Geometry: final body of the model. Coordinates: model frame, mm. Face numbers are marked on the shaded views. A direction names the side the tool comes from. Coordinates: 2 decimals unless noted, no trailing zeros. Write each loop counter-clockwise with the first axis right and the second up, starting at its lowest first coordinate (ties: lowest second). Pieces come first, ordered by that corner, then holes. Notation, with made-up numbers: (63, 4) - (92, 4) arc R18 cw to (92, 8) - close; hole circle Ø5 at (57, -26). An arc over 180 degrees is marked (long way). Put each result on its own line as item: value.
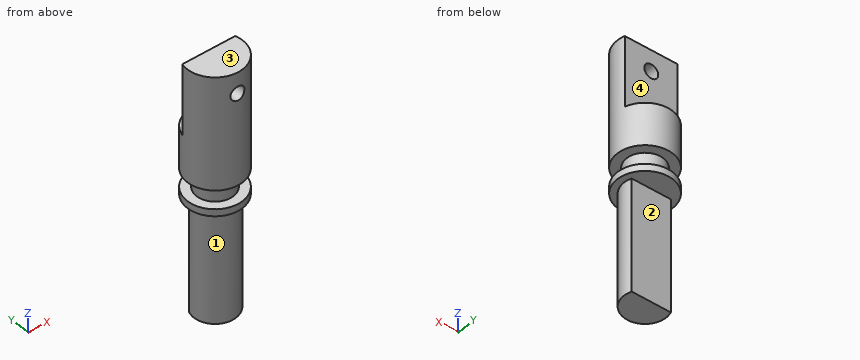
Autodesk Inventor part; units mm, degrees
ref_plane "YZ Plane" through (0, 0, 0) normal (1, 0, 0) x (0, 1, 0)
ref_plane "XZ Plane" through (0, 0, 0) normal (0, 1, 0) x (-1, 0, 0)
ref_plane "XY Plane" through (0, 0, 0) normal (0, 0, 1) x (1, 0, 0)
sketch "Sketch1" plane through (0, 0, 0) normal (0, 1, 0) x (-1, 0, 0)
  line L0 (0, 0) -> (-2.8001, 0)
  line L1 (-2.8001, 0) -> (-3.937, 0)
  line L2 (-3.937, 0) -> (-3.937, -16)
  line L3 (-3.937, -16) -> (-2.6225, -16)
  line L4 (-2.6225, -16) -> (-2.6225, -18.6416)
  line L5 (-2.6225, -18.6416) -> (-3.937, -18.6416)
  line L6 (-3.937, -18.6416) -> (-3.937, -19.6416)
  line L7 (-2.8001, 0) -> (0, 0)
  line L8 (-2.8001, 0) -> (0, 0)
  line L9 (-3.937, -19.6416) -> (-3, -19.6416)
  line L10 (-3, -19.6416) -> (-3, -35.6416)
  line L11 (-3, -35.6416) -> (0, -35.6416)
  line L12 (0, -35.6416) -> (0, 0)
  dimension "d1" = 0
  dimension "d2" = 16
  dimension "d3" = 2.6416
  dimension "d6" = 3.937
  dimension "d8" = 3
  dimension "d13" = 1
  dimension "d29" = 2.6225
  dimension "d30" = 16
revolve "Revolution1" add sketch "Sketch1" angle 360 about axis through (0, 0, -35.6416) along (0, 0, 1)
thread "Thread1"
sketch "Sketch3" plane through (0, 0, 0) normal (0, 0, 1) x (1, 0, 0)
  circle A0 centre (0, 0) radius 3.937
  line L0 (-3.033, -2.5101) -> (3.033, -2.5101)
  line L1 (-3.7908, 1.063) -> (3.7908, 1.063)
  arc A1 (3.033, -2.5101) -> (3.7908, 1.063) centre (0, 0) ccw
  arc A2 (-3.7908, 1.063) -> (-3.033, -2.5101) centre (0, 0) ccw
  point P0 (0, 0)
  dimension "d36" = 5
extrude "Extrusion1" cut sketch "Sketch3" against normal blind 10 contours L1 A0
sketch "Sketch4" plane through (-3.7908, 1.063, 0) normal (0, 1, 0) x (1, 0, 0)
  circle A0 centre (3.7908, 3) radius 1
  point P0 (3.7908, 0)
  dimension "d23" = 2
  dimension "d24" = 3
extrude "Extrusion2" cut sketch "Sketch4" against normal blind 10
thread "Thread2"
sketch "Sketch5" plane through (0, 0, -35.6416) normal (0, 0, -1) x (-1, 0, 0)
  circle A0 centre (0, 0) radius 3.937
  line L0 (-3.7908, 1.063) -> (5.4234, 1.063)
  line L1 (5.4234, 1.063) -> (5.4234, 3.7958)
  line L2 (5.4234, 3.7958) -> (-3.7908, 3.7958)
  line L3 (-3.7908, 3.7958) -> (-3.7908, 1.063)
  point P0 (0, 0)
  dimension "d33" = 5
extrude "Extrusion3" cut sketch "Sketch5" against normal blind 16 contours L3 L2 A0 | A0 L2 L0 | A0 L2 L1 L0
properties part number "rod"
1. Section query D-D (z = -22). Return loops of the section in (x, y).
Answer below:
outline: (-2.81, 1.06) arc R3 ccw (long way) to (2.81, 1.06) - close
2. Section query C-C (z = -3.5). Return loops of the section in (x, y).
Answer below:
outline: (-3.79, 1.06) arc R3.94 ccw to (-0.87, -3.84) - (-0.87, 1.06) - close; (0.87, -3.84) arc R3.94 ccw to (3.79, 1.06) - (0.87, 1.06) - close
3. Pin query (flat end, axial travel): pin 1 Ø2.5 at (x, y) = (0.5, 2) entering from -Z; pin 2 Ø2 at (y, z) = (-1, -20.5) entering from -X; pin 3 Ø0.9 at (x, y) = (-1, 2) entering from +Z; pin 4 Ø1.7 at (x, z) = (-0.5, -30) entering from +Y. Return the tip coordinate at first contact, or that it passes through.
Answer below:
pin 1: stops at z = -35.64
pin 2: stops at x = -3.91
pin 3: stops at z = -10
pin 4: stops at y = 1.06
4. Ray query, probe 1 along Z at (x, y) = (0, -2.05); probe 2 along X at (y, z) = (0, -3); probe 3 along Z at (x, y) = (-2.5, -2.25). Return the intervals inside material, ascending. Write a range as from..to.
Answer below:
probe 1: z = -35.64..-4, -2..0
probe 2: x = -3.94..-1, 1..3.94
probe 3: z = -19.64..-18.64, -16..0
5. Set-up query: the marked faces 1, 2, 3 and 4. Return all of +Z, -Z, +X, -X, +Y, -Y with unobstructed straight access to the full face (end or side cutting, diameter ignored); none if empty.
Answer below:
face 1: -Z
face 2: -Z, +X, -X, +Y
face 3: +Z, +X, -X, +Y, -Y
face 4: +Z, +X, -X, +Y
6. Section query B-B (x = 0). Return loops of the section in (y, z), then the cut area to 3 significant figures.
Answer below:
outline: (-3.94, -19.64) - (-3, -19.64) - (-3, -35.64) - (1.06, -35.64) - (1.06, -19.64) - (3.94, -19.64) - (3.94, -18.64) - (2.62, -18.64) - (2.62, -16) - (3.94, -16) - (3.94, -10) - (1.06, -10) - (1.06, -4) - (-3.94, -4) - (-3.94, -16) - (-2.62, -16) - (-2.62, -18.64) - (-3.94, -18.64) - close; (-3.94, -2) - (1.06, -2) - (1.06, 0) - (-3.94, 0) - close
area: 174 mm²
7. Section query A-A (y = 0). Return loops of the section in (x, z).
Answer below:
outline: (-3.94, -19.64) - (-3, -19.64) - (-3, -35.64) - (3, -35.64) - (3, -19.64) - (3.94, -19.64) - (3.94, -18.64) - (2.62, -18.64) - (2.62, -16) - (3.94, -16) - (3.94, 0) - (-3.94, 0) - (-3.94, -16) - (-2.62, -16) - (-2.62, -18.64) - (-3.94, -18.64) - close; hole circle Ø2 at (0, -3)
